Input: part model. Units: mm. Frame: model coordinates. A direction names the side the tool comes from. Round coordinates to 2 decimals unless told otherwise and drop trailing zeros. Loops run counter-clockwise (first coordinate to the right, second up) from the corner with the lowest first, then second, coordinate; pieces in that order, holes last.
1) Section A-A, the plane x = -4. Return loops of the section in (y, z), and give its area (3 significant figures).
2) Draft query along Y for faces 1 (the face through (0, 22, -9)), 2 (the face through (0, -22, -8)), 3 (the face through (17.5, 0, 3)), 4 (the face through (12, 0, 0)). Return one class per face: pulls with the +Y half, pulls with the -Y half, needs draft (parallel to the pull), parting line crosses it, or undercut.
3) Ray query, line 1 along Y through (x, z) = (0, 2); line 2 along Y through (x, z) = (2.5, -15); line 3 along Z through (x, y) = (-10, -20). Return the intervals inside material, ascending.
4) First-contact query: pin 1 (3 mm diameter, centred on x = -10, z = -8, fed in from -Y). Flat tip, straight axial feed; report the tip coordinate or a pass-through.
5) Section C-C, the plane y = 10. Return loops of the section in (x, z), and give its area (3 significant figures).
6) Section D-D, the plane x = -10. Return loops of the section in (y, z).
7) Section B-B, the plane z = -18. Return loops of the section in (x, y).
8) Access query for faces 5 (the face through (-10, -20, -10)), 6 (the face through (0, -18, -10)), 7 (the face through (0, -11, 2)). Directions: +Z, -Z, +X, -X, +Y, -Y. A direction counts if a zero-diameter tool reaches every point of the face in a straight line with its end or side. Return the directions, or none.
from build123d import *

# Parameters (mm, degrees)
SKETCH_1_R      = 1.2
SKETCH_1_W      = 22
SKETCH_1_H      = 22
EXTRUDE_1_DEPTH = 4
SKETCH_2_W      = 35
SKETCH_2_H      = 25
SKETCH_2_R      = 2
EXTRUDE_2_DEPTH = 4
SKETCH_3_W      = 35
SKETCH_3_H      = 25
EXTRUDE_3_DEPTH = 4


with BuildPart() as part:
    # 草图1 → 凸台-拉伸1 (new body)
    with BuildSketch(Plane.XY):
        Polygon((17.5, 0), (17.5, -18), (-17.5, -18), (-17.5, 0), (-17.5, 18), (17.5, 18), align=None)
        with Locations((0, 14.5)):
            Circle(SKETCH_1_R, mode=Mode.SUBTRACT)
        with Locations((14.5, 0)):
            Circle(SKETCH_1_R, mode=Mode.SUBTRACT)
        with Locations((0, -14.5)):
            Circle(SKETCH_1_R, mode=Mode.SUBTRACT)
        with Locations((-14.5, 0)):
            Circle(SKETCH_1_R, mode=Mode.SUBTRACT)
        Rectangle(SKETCH_1_W, SKETCH_1_H, mode=Mode.SUBTRACT)
    extrude(amount=EXTRUDE_1_DEPTH)

    # 草图2 → 凸台-拉伸2 (add)
    with BuildSketch(Plane.XZ.offset(18)):
        with Locations((0, -8.5)):
            Rectangle(SKETCH_2_W, SKETCH_2_H)
        with Locations((10, -8)):
            Circle(SKETCH_2_R, mode=Mode.SUBTRACT)
        with Locations((0, -15)):
            Circle(SKETCH_2_R, mode=Mode.SUBTRACT)
        with Locations(Location((-10, -8, 0), (0, 0, 180))):
            Circle(SKETCH_2_R, mode=Mode.SUBTRACT)
    extrude(amount=EXTRUDE_2_DEPTH)

    # 草图3 → 凸台-拉伸3 (add)
    with BuildSketch(Plane(origin=(0, 18, 0), x_dir=(1, 0, 0), z_dir=(0, 1, 0))):
        with Locations((0, 8.5)):
            Rectangle(SKETCH_3_W, SKETCH_3_H)
    extrude(amount=EXTRUDE_3_DEPTH)


solid = part.part
Final values:
1. outline: (-22, -21) - (-18, -21) - (-18, 0) - (-11, 0) - (-11, 4) - (-22, 4) - close; (11, 0) - (18, 0) - (18, -21) - (22, -21) - (22, 4) - (11, 4) - close
1. area: 256 mm2
2. face 1: pulls with the +Y half
2. face 2: pulls with the -Y half
2. face 3: needs draft
2. face 4: undercut
3. line 1: y = -22 to -15.7, -13.3 to -11, 11 to 13.3, 15.7 to 22
3. line 2: y = -22 to -18, 18 to 22
3. line 3: z = -21 to -10, -6 to 4
4. pin 1: stops at y = 18
5. outline: (-17.5, 0) - (-11, 0) - (-11, 4) - (-17.5, 4) - close; (11, 0) - (17.5, 0) - (17.5, 4) - (11, 4) - close
5. area: 52.0 mm2
6. outline: (-22, -21) - (-18, -21) - (-18, -10) - (-22, -10) - close; (-22, -6) - (-18, -6) - (-18, 0) - (-11, 0) - (-11, 4) - (-22, 4) - close; (11, 0) - (18, 0) - (18, -21) - (22, -21) - (22, 4) - (11, 4) - close
7. outline: (-17.5, -22) - (17.5, -22) - (17.5, -18) - (-17.5, -18) - close; (-17.5, 18) - (17.5, 18) - (17.5, 22) - (-17.5, 22) - close
8. face 5: -Y
8. face 6: -Z, +X, -X
8. face 7: +Z, -Z
